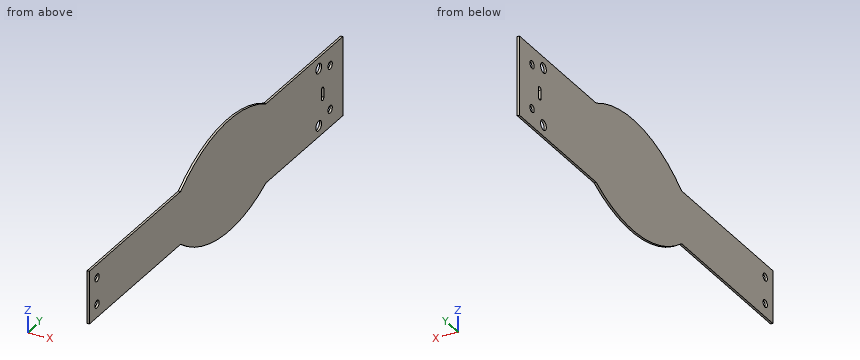
```python
from build123d import *

# Parameters (mm, degrees)
BOSS_EXTRUDE1_DEPTH  = 1
M3_CLEARANCE_HOLE1_D = 3.4
M4_CLEARANCE_HOLE1_D = 4.5
CUT_EXTRUDE1_DEPTH   = 202.589376266
M3_CLEARANCE_HOLE2_D = 3.4


with BuildPart() as part:
    # Sketch1 → Boss-Extrude1 (new body)
    with BuildSketch(Plane(origin=(0, 0, 0), x_dir=(0, 0, -1), z_dir=(1, 0, 0))):
        with BuildLine():
            Line((12, -200), (12, -128))
            ThreePointArc((12, -128), (25, -95.198992339), (18, -60.617116977))
            Line((18, -60.617116977), (18, 0))
            Line((18, 0), (-18, 0))
            Line((-18, 0), (-18, -60.617116977))
            ThreePointArc((-18, -60.617116977), (-25, -95.198992339), (-12, -128))
            Line((-12, -128), (-12, -200))
            Line((-12, -200), (12, -200))
        make_face()
    extrude(amount=BOSS_EXTRUDE1_DEPTH)

    # M3 Clearance Hole1 (through all)
    with Locations(Plane.ZY):
        with Locations((10, -10), (-10, -10)):
            Hole(M3_CLEARANCE_HOLE1_D / 2)

    # M4 Clearance Hole1 (through all)
    with Locations(Plane.ZY):
        with Locations((-13, -19), (13, -19)):
            Hole(M4_CLEARANCE_HOLE1_D / 2)

    # Sketch10 → Cut-Extrude1 (cut, through all)
    with BuildSketch(Plane(origin=(1, 0, 0), x_dir=(0, 0, -1), z_dir=(1, 0, 0))):
        with BuildLine():
            Line((-2, -15), (2, -15))
            ThreePointArc((2, -15), (3, -16), (2, -17))
            Line((2, -17), (-2, -17))
            ThreePointArc((-2, -17), (-3, -16), (-2, -15))
        make_face()
    extrude(amount=-CUT_EXTRUDE1_DEPTH, mode=Mode.SUBTRACT)

    # M3 Clearance Hole2 (through all)
    with Locations(Plane(origin=(1, 0, 0), x_dir=(0, 0, -1), z_dir=(1, 0, 0))):
        with Locations((-6, -194), (6, -194)):
            Hole(M3_CLEARANCE_HOLE2_D / 2)


solid = part.part
```
The listing builds one solid part. Answer for the finished solid, in the listing's coordinates (mm). Coordinates: 2 decimals unless noted, no trailing zeros. Loops run counter-clockwise (first coordinate to the right, second up) from the corner with the lowest first, then second, coordinate; pieces in that order, holes last. Notation, with made-up numbers: (31, 48.25) - (44, 48.25) arc R31 cw to (44, 87.25) - close; hole circle Ø10 at (-10, 5.25). An arc over 180 degrees is marked (long way). Use a Markdown table: item, result. Add a question column.
1) The part is cut by section D-D, the plane y = -130. Give the vertices of the cut face in (x, z), and give its area (3 significant figures).
2) Find the intervals of material crossed by line 1 (Z direction, x = 0.8, y = -194); line 2 (Y direction, x = 0.6, z = -10); line 3 (Y direction, x = 0.3, z = 1), in increasing order.
3) The part is cut by section B-B, the plane x = 0.8. Give the vertices of the cut face in (y, z).
4) The part is cut by section C-C, the plane y = -194. Give the vertices of the cut face in (x, z).
5) The part is cut by section A-A, the plane y = -19. Give the vertices of the cut face in (x, z), and give its area (3 significant figures).
6) Given pin 1 (4 mm diameter, centred on y = -194, z = -6, fed in from -X); pin 2 (0.5 mm diameter, centred on x = 0.5, y = -173, fed in from +Z); pin 3 (0.5 mm diameter, centred on x = 0.5, y = -24.5, fed in from -Z), each flat-ended and moving along its own axis, determine where each tip first touches the part or whether it passes through.
Here are the results:
| question | item | result |
|---|---|---|
| 1 | outline | (0, -12) - (1, -12) - (1, 12) - (0, 12) - close |
| 1 | area | 24.0 mm^2 |
| 2 | line 1 | z = -12 to -7.7, -4.3 to 4.3, 7.7 to 12 |
| 2 | line 2 | y = -200 to -11.7, -8.3 to 0 |
| 2 | line 3 | y = -200 to -17, -15 to 0 |
| 3 | outline | (-200, -12) - (-128, -12) arc R62 ccw to (-60.62, -18) - (0, -18) - (0, 18) - (-60.62, 18) arc R62 ccw to (-128, 12) - (-200, 12) - close; hole circle Ø3.4 at (-194, -6); hole circle Ø3.4 at (-194, 6); hole circle Ø4.5 at (-19, -13); hole circle Ø4.5 at (-19, 13); hole (-17, -2) arc R1 ccw to (-15, -2) - (-15, 2) arc R1 ccw to (-17, 2) - close; hole circle Ø3.4 at (-10, -10); hole circle Ø3.4 at (-10, 10) |
| 4 | outline | (0, -12) - (1, -12) - (1, -7.7) - (0, -7.7) - close; (0, -4.3) - (1, -4.3) - (1, 4.3) - (0, 4.3) - close; (0, 7.7) - (1, 7.7) - (1, 12) - (0, 12) - close |
| 5 | outline | (0, -18) - (1, -18) - (1, -15.25) - (0, -15.25) - close; (0, -10.75) - (1, -10.75) - (1, 10.75) - (0, 10.75) - close; (0, 15.25) - (1, 15.25) - (1, 18) - (0, 18) - close |
| 5 | area | 27.0 mm^2 |
| 6 | pin 1 | stops at x = 0 |
| 6 | pin 2 | stops at z = 12 |
| 6 | pin 3 | stops at z = -18 |
